For this review, take the finished solid that the model builds, in its own axes (mm). Face numbers are marked on the shaded views. Coordinates: 2 decimals unless noted, no trailing zeros. Write each loop counter-clockwise with the first axis right and the second up, starting at its lowest first coordinate (ties: lowest second). Pieces come first, ordered by that corner, then holes. Notation, with made-up numbers: (31, -23.75) -> (76, -23.75) arc R7 ccw to (76, -18.75) -> close; hole circle Ø6 at (60, -17). An arc over 180 degrees is marked (long way). Put each result on its own line as item: value. Start each with the question number.
Item 1: The part is to be moulded in two halves that separate along Z. For the marked faces 1, 2 and 3, say which applies: +Z half, -Z half, draft (parallel to the pull), parting line (faces both ways), or undercut.
Item 2: Consider section B-B on x = 0. Give the boundary of the cut face in (y, z).
Item 3: Consider section C-C on y = 12.75. Give the boundary of the cut face in (x, z).
Item 4: Insertion check: P1, Ø3, axis at y = 3, z = -2, coming from the -X side. The pin has a flat end and moves straight along its axis. Give the tip position at first contact, or say it passes through.
Item 5: Consider section A-A on z = 0. Give the boundary of the cut face in (x, y), and give its area (3 significant figures).
Item 6: To check wall thickness, follow L1, parallel to Z at x = 0, y = 15; L2, parallel to Z at x = 0.55, y = 2.5; L3, parallel to X at y = 12.5, z = 0.6. State the ranges of each line that lie inside material, in increasing order.
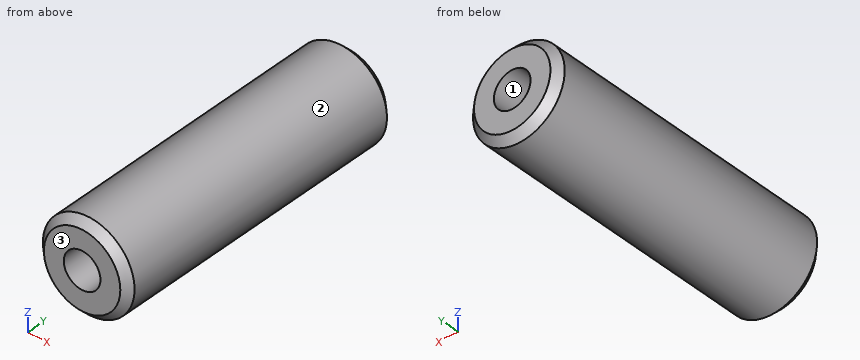
```python
from build123d import *

# Parameters (mm, degrees)
F0_R     = 3
F1_DEPTH = 20
F2_D     = 2.4
F3_SIZE  = 0.5


with BuildPart() as f1:
    # F0 (on Front) → F1 (new body)
    with BuildSketch(Plane.XZ):
        Circle(F0_R)
    extrude(amount=-F1_DEPTH)

    # F2 (through all)
    with Locations(Plane.XZ):
        with Locations((0, 0)):
            Hole(F2_D / 2)

    # F3
    f3_edges = [f1.edges().sort_by_distance(p)[0] for p in [
        (-3, 0, 0),
        (-3, 20, 0),
    ]]
    chamfer(f3_edges, length=F3_SIZE)


solid = f1.part
```
Return value:
1. face 1: undercut
1. face 2: parting line
1. face 3: draft
2. outline: (0, -2.5) -> (0.5, -3) -> (19.5, -3) -> (20, -2.5) -> (20, -1.2) -> (0, -1.2) -> close; (0, 1.2) -> (20, 1.2) -> (20, 2.5) -> (19.5, 3) -> (0.5, 3) -> (0, 2.5) -> close
3. outline: circle Ø6 at (0, 0); hole circle Ø2.4 at (0, 0)
4. P1: x = -2.96
5. outline: (-3, 0.5) -> (-2.5, 0) -> (-1.2, 0) -> (-1.2, 20) -> (-2.5, 20) -> (-3, 19.5) -> close; (1.2, 0) -> (2.5, 0) -> (3, 0.5) -> (3, 19.5) -> (2.5, 20) -> (1.2, 20) -> close
5. area: 71.5 mm^2
6. L1: -3 to -1.2, 1.2 to 3
6. L2: -2.95 to -1.07, 1.07 to 2.95
6. L3: -2.94 to -1.04, 1.04 to 2.94
